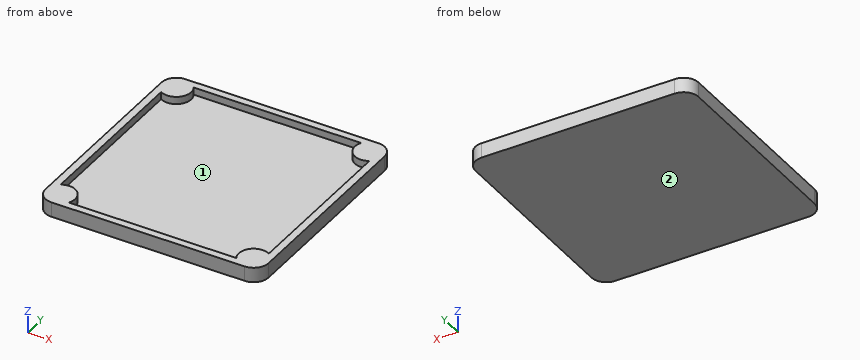
```python
from build123d import *

# Parameters (mm, degrees)
F0_W     = 30
F0_H     = 30
F1_DEPTH = 2
F3_DEPTH = 1
F5_R     = 1.5
F6_DEPTH = 1.5
F7_R     = 2


with BuildPart() as f1:
    # F0 (on Top) → F1 (new body)
    with BuildSketch(Plane.XY):
        Rectangle(F0_W, F0_H)
    extrude(amount=F1_DEPTH)

    # F2 (on face) → F3 (cut)
    with BuildSketch(Plane.XY.offset(2)):
        with BuildLine():
            ThreePointArc((-11.267949, 14), (-11.585786, 11.585786), (-14, 11.267949))
            Line((-14, 11.267949), (-14, -11.267949))
            ThreePointArc((-14, -11.267949), (-11.585786, -11.585786), (-11.267949, -14))
            Line((-11.267949, -14), (11.267949, -14))
            ThreePointArc((11.267949, -14), (11.585786, -11.585786), (14, -11.267949))
            Line((14, -11.267949), (14, 11.267949))
            ThreePointArc((14, 11.267949), (11.585786, 11.585786), (11.267949, 14))
            Line((11.267949, 14), (-11.267949, 14))
        make_face()
    extrude(amount=-F3_DEPTH, mode=Mode.SUBTRACT)

    # F5 (on offset) → F6 (cut)
    with BuildSketch(Plane.XY.offset(1.8)):
        with Locations((-13, 13)):
            Circle(F5_R)
        with Locations((13, 13)):
            Circle(F5_R)
        with Locations((-13, -13)):
            Circle(F5_R)
        with Locations((13, -13)):
            Circle(F5_R)
    extrude(amount=-F6_DEPTH, mode=Mode.SUBTRACT)

    # F7
    f7_edges = [f1.edges().sort_by_distance(p)[0] for p in [
        (-15, 15, 1),
        (-15, -15, 1),
        (15, -15, 1),
        (15, 15, 1),
    ]]
    fillet(f7_edges, radius=F7_R)


solid = f1.part
```
Read the model definition and answer for the solid it produces. Units are mm, in the model's axes. Face numbers are marked on the shaded views. Give positions to 0.01 mm unless a question says otherwise; leave off trailing zeros. Order: outer loops, then holes, each group sorted by start corner. A loop starts at its lowest first (then second) coordinate and runs counter-clockwise, first axis right, second up. Notation, with made-up numbers: (54, 84) -> (88, 84) arc R21 cw to (88, 92) -> close; hole circle Ø7 at (-29.75, 49.5). An arc over 180 degrees is marked (long way). One line per item, written item: value. Start each with the question number.
(1) For a pull along X with two mould halves and no side action, classify the marked faces 1 and 2 as released by +X, released by -X, zero draft, split by the parting line, or undercut.
(2) A flat-ended cylindrical pin translates along its axis: P1, Ø6, axis at x = 0, y = -5.5, coming from the +Z side. Find the tip coordinate at first contact, or state that the pin passes through.
(3) Straight lines are drawn through the part: L1, parallel to Y at x = -13, z = 1.55; L2, parallel to Y at x = 13, z = 0.85; L3, parallel to Y at x = 9.75, z = 1.25. For each, find the intervals that lie inside material, in ascending order.
(4) The part is cut by section A-A (x = 5). Determine the outline of the cut face in (y, z), and give its area (3 significant figures).
Taken from the geometry:
1. face 1: undercut
1. face 2: zero draft
2. P1: z = 1
3. L1: -15 to -14.5, -11.5 to -11, 11 to 11.5, 14.5 to 15
3. L2: -15 to -14.5, -11.5 to 11.5, 14.5 to 15
3. L3: -15 to -14, 14 to 15
4. outline: (-15, 0) -> (15, 0) -> (15, 2) -> (14, 2) -> (14, 1) -> (-14, 1) -> (-14, 2) -> (-15, 2) -> close
4. area: 32.0 mm^2
